```python
from build123d import *

# Parameters (mm, degrees)
SKETCH1_W           = 156.7
SKETCH1_H           = 140
BOSS_EXTRUDE1_DEPTH = 3
SKETCH2_W           = 126.7
SKETCH2_H           = 20
CUT_EXTRUDE1_DEPTH  = 106.108146687
FILLET1_R           = 2
SKETCH3_W           = 3.7
SKETCH3_H           = 28
CUT_EXTRUDE2_DEPTH  = 106.108146687
SKETCH4_W           = 52.3
SKETCH4_H           = 5
BOSS_EXTRUDE2_DEPTH = 3
SKETCH5_R           = 1
CUT_EXTRUDE3_DEPTH  = 109.502177398
SKETCH6_R           = 2
CUT_EXTRUDE4_DEPTH  = 109.502177398


with BuildPart() as part:
    # Sketch1 → Boss-Extrude1 (new body)
    with BuildSketch(Plane.XY):
        Rectangle(SKETCH1_W, SKETCH1_H)
    extrude(amount=BOSS_EXTRUDE1_DEPTH)

    # Sketch2 → Cut-Extrude1 (cut, through all)
    with BuildSketch(Plane.XY.offset(3)):
        with Locations((0, -50)):
            Rectangle(SKETCH2_W, SKETCH2_H)
        Polygon((-62.25, 45), (-62.25, -20), (-12.633333333, 12.5), align=None)
        Polygon((0, 4.22489083), (-52.25, -30), (52.25, -30), align=None)
        Polygon((-52.25, 55), (0, 20.77510917), (52.25, 55), align=None)
        Polygon((62.25, 45), (12.633333333, 12.5), (62.25, -20), align=None)
    extrude(amount=-CUT_EXTRUDE1_DEPTH, mode=Mode.SUBTRACT)

    # Fillet1
    fillet1_edges = [part.edges().sort_by_distance(p)[0] for p in [
        (63.35, -60, 1.5),
        (-63.35, -60, 1.5),
        (-63.35, -40, 1.5),
        (63.35, -40, 1.5),
        (-12.633333333, 12.5, 1.5),
        (-62.25, -20, 1.5),
        (-62.25, 45, 1.5),
        (-52.25, -30, 1.5),
        (0, 4.22489083, 1.5),
        (52.25, -30, 1.5),
        (52.25, 55, 1.5),
        (0, 20.77510917, 1.5),
        (-52.25, 55, 1.5),
        (12.633333333, 12.5, 1.5),
        (62.25, 45, 1.5),
        (62.25, -20, 1.5),
    ]]
    fillet(fillet1_edges, radius=FILLET1_R)

    # Sketch3 → Cut-Extrude2 (cut, through all)
    with BuildSketch(Plane.XY.offset(3)):
        with Locations((-76.5, 28)):
            Rectangle(SKETCH3_W, SKETCH3_H)
        with Locations((-76.5, -28)):
            Rectangle(SKETCH3_W, SKETCH3_H)
        with Locations((76.5, 56)):
            Rectangle(SKETCH3_W, SKETCH3_H)
        with Locations((76.5, 0)):
            Rectangle(SKETCH3_W, SKETCH3_H)
        with Locations((76.5, -56)):
            Rectangle(SKETCH3_W, SKETCH3_H)
    extrude(amount=-CUT_EXTRUDE2_DEPTH, mode=Mode.SUBTRACT)

    # Sketch4 → Boss-Extrude2 (add)
    with BuildSketch(Plane.XY.offset(3)):
        with Locations((0, -72.5)):
            Rectangle(SKETCH4_W, SKETCH4_H)
    extrude(amount=-BOSS_EXTRUDE2_DEPTH)

    # Sketch5 → Cut-Extrude3 (cut, through all)
    with BuildSketch(Plane.XY.offset(3)):
        with Locations((-74.65, 42)):
            Circle(SKETCH5_R)
        with Locations((-74.65, 14)):
            Circle(SKETCH5_R)
        with Locations((-74.65, -14)):
            Circle(SKETCH5_R)
        with Locations((-74.65, -42)):
            Circle(SKETCH5_R)
        with Locations((-26.15, -70)):
            Circle(SKETCH5_R)
        with Locations((26.15, -70)):
            Circle(SKETCH5_R)
        with Locations((74.65, -42)):
            Circle(SKETCH5_R)
        with Locations((74.65, -14)):
            Circle(SKETCH5_R)
        with Locations((74.65, 42)):
            Circle(SKETCH5_R)
        with Locations((74.65, 14)):
            Circle(SKETCH5_R)
    extrude(amount=-CUT_EXTRUDE3_DEPTH, mode=Mode.SUBTRACT)

    # Sketch6 → Cut-Extrude4 (cut, through all)
    with BuildSketch(Plane(origin=(0, 0, 0), x_dir=(-1, 0, 0), z_dir=(0, 0, -1))):
        with Locations((-62.25, 62.5)):
            Circle(SKETCH6_R)
    extrude(amount=-CUT_EXTRUDE4_DEPTH, mode=Mode.SUBTRACT)


solid = part.part
```
Design review of the part built by this model. Coordinates are the model's own, in mm. A direction names the side the tool comes from. Coordinates: 2 decimals unless noted, no trailing zeros. Loops run counter-clockwise (first coordinate to the right, second up) from the corner with the lowest first, then second, coordinate; pieces in that order, holes last. Notation, with made-up numbers: (-8.5, 79.25) - (5.5, 79.25) arc R8 ccw to (5.5, 92.25) - close; hole circle Ø7 at (-7.5, -27.5). An arc over 180 degrees is marked (long way). Use CSV: the item, a comma, the result in double quotes. Start each with the question number.
1) Consider section D-D on x = -38. Write out the cut boundary in (y, z).
2) Tool access review of faces 4 (the flat face through (23.55, 36.2, 1.52)), 5 (the flat face through (16, -1, 3)): name each direction out of +Z, -Z, +X, -X, +Y, -Y from which nothing blocks a thin tool from reaching the whole face with its end or side.
3) The part is to be moulded in two halves that separate along Y. For faces 1 (the flat face through (24.19, -11.62, 1.52)), 2 (the flat face through (-36.86, 28.37, 1.52)), 3 (the flat face through (16, -1, 0)), say which applies: +Y half, -Y half, draft (parallel to the pull), parting line (faces both ways), or undercut.
4) Wall thickness on L1, parallel to Y at x = -33.5, z = 1.45; L2, parallel to X at y = -4.5, z = 1.75; L3, parallel to Y at x = 19, z = 2.6: over which ranges is each line inside the solid? List them lowest first. Write a range as from..to.
5) Consider section C-C on y = -7.5. Write out the cut boundary in (x, z).
6) Consider section A-A on y = 62.5. Write out the cut boundary in (x, z).
7) Consider section B-B on x = 56.5. Write out the cut boundary in (y, z).
8) For pin 1 Ø1.2 at (x, y) = (74.65, -42) entering from -Z; pin 2 Ø0.8 at (x, z) = (77, 1) entering from -Y; pin 3 Ø0.9 at (y, z) = (-54.5, 1) entering from +X; pin 4 Ø0.9 at (x, z) = (41.5, 2) entering from -Y, all flat-tipped, find the tip position at first contact; note any pin that passes through.
Geometry says:
1,outline,"(-70, 0) - (-60, 0) - (-60, 3) - (-70, 3) - close; (-40, 0) - (-30, 0) - (-30, 3) - (-40, 3) - close; (-20.67, 0) - (-4.12, 0) - (-4.12, 3) - (-20.67, 3) - close; (29.12, 0) - (45.67, 0) - (45.67, 3) - (29.12, 3) - close; (55, 0) - (70, 0) - (70, 3) - (55, 3) - close"
2,face 4,"+Z, -Z"
2,face 5,"+Z, +X, -X, +Y, -Y"
3,face 1,"undercut"
3,face 2,"undercut"
3,face 3,"draft"
4,L1,"-70..-60, -40..-30, -17.72..-1.17, 26.17..42.72, 55..70"
4,L2,"-78.35..-62.25, -38.59..-13.32, 13.32..38.59, 62.25..74.65"
4,L3,"-75..-60, -40..-30, -8.22..8.33, 16.67..33.22, 55..70"
5,outline,"(-78.35, 0) - (-62.25, 0) - (-62.25, 3) - (-78.35, 3) - close; (-43.17, 0) - (-17.9, 0) - (-17.9, 3) - (-43.17, 3) - close; (17.9, 0) - (43.17, 0) - (43.17, 3) - (17.9, 3) - close; (62.25, 0) - (74.65, 0) - (74.65, 3) - (62.25, 3) - close"
6,outline,"(-78.35, 0) - (60.25, 0) - (60.25, 3) - (-78.35, 3) - close; (64.25, 0) - (74.65, 0) - (74.65, 3) - (64.25, 3) - close"
7,outline,"(-70, 0) - (-60, 0) - (-60, 3) - (-70, 3) - close; (-40, 0) - (-16.23, 0) - (-16.23, 3) - (-40, 3) - close; (41.23, 0) - (70, 0) - (70, 3) - (41.23, 3) - close"
8,pin 1,"through"
8,pin 2,"y = -42"
8,pin 3,"x = 74.65"
8,pin 4,"y = -70"
